from build123d import *

# Parameters (mm, degrees)
EXTRUDE_1_DEPTH     = 5
SKETCH_18_W         = 75
SKETCH_18_H         = 10
EXTRUDE_2_DEPTH     = 30
SKETCH_19_R         = 2.5
CUT_EXTRUDE_3_DEPTH = 85.889634232
EXTRUDE_3_DEPTH     = 10
SKETCH_21_R         = 2.5
CUT_EXTRUDE_4_DEPTH = 137.267200749


with BuildPart() as part:
    # ｽｹｯﾁ1 → ﾎﾞｽ - 押し出し1 (new body)
    with BuildSketch(Plane(origin=(0, 0, 0), x_dir=(1, 0, 0), z_dir=(0, 1, 0))):
        with BuildLine():
            Line((-37.5, 0), (-37.5, -70))
            Line((-37.5, -70), (37.5, -70))
            Line((37.5, -70), (37.5, 0))
            ThreePointArc((37.5, 0), (0, 37.5), (-37.5, 0))
        make_face()
    extrude(amount=EXTRUDE_1_DEPTH)

    # ｽｹｯﾁ18 → ﾎﾞｽ - 押し出し2 (add)
    with BuildSketch(Plane(origin=(0, 5, 0), x_dir=(1, 0, 0), z_dir=(0, 1, 0))):
        with Locations((0, -65)):
            Rectangle(SKETCH_18_W, SKETCH_18_H)
    extrude(amount=EXTRUDE_2_DEPTH)

    # ｽｹｯﾁ19 → ｶｯﾄ - 押し出し3 (cut, through all)
    with BuildSketch(Plane(origin=(0, 5, 0), x_dir=(1, 0, 0), z_dir=(0, 1, 0))):
        with Locations(Location((0, 31.5, 0), (0, 0, 270))):
            Circle(SKETCH_19_R)
        with Locations(Location((0, -31.5, 0), (0, 0, 90))):
            Circle(SKETCH_19_R)
    extrude(amount=-CUT_EXTRUDE_3_DEPTH, mode=Mode.SUBTRACT)

    # ｽｹｯﾁ20 → ﾎﾞｽ - 押し出し3 (add)
    with BuildSketch(Plane.XY.offset(70)):
        with BuildLine():
            Line((-37.5, 50), (-37.5, 35))
            Line((-37.5, 35), (37.5, 35))
            Line((37.5, 35), (37.5, 50))
            ThreePointArc((37.5, 50), (0, 87.5), (-37.5, 50))
        make_face()
    extrude(amount=-EXTRUDE_3_DEPTH)

    # ｽｹｯﾁ21 → ｶｯﾄ - 押し出し4 (cut, through all)
    with BuildSketch(Plane(origin=(0, 0, 60), x_dir=(-1, 0, 0), z_dir=(0, 0, -1))):
        with Locations((0, 81.5)):
            Circle(SKETCH_21_R)
        with Locations(Location((0, 18.5, 0), (0, 0, 180))):
            Circle(SKETCH_21_R)
    extrude(amount=-CUT_EXTRUDE_4_DEPTH, mode=Mode.SUBTRACT)


solid = part.part
Verification items for the finished model (mm, model axes). A direction names the side the tool comes from. Coordinates: 2 decimals unless noted, no trailing zeros. Write each loop counter-clockwise with the first axis right and the second up, starting at its lowest first coordinate (ties: lowest second). Pieces come first, ordered by that corner, then holes. Notation, with made-up numbers: (53, 66.25) -> (69, 66.25) arc R14 cw to (69, 89.25) -> close; hole circle Ø6 at (-37, 39.25). An arc over 180 degrees is marked (long way). One line per item, written item: value. Start each with the question number.
Q1. Mould release check, pull along Z, two halves, no side actions. Record for faces 1 (the cylindrical face through (0, 3, -34)), 2 (the flat face through (37.5, 4.5, 50.7)), 3 (the flat face through (-1, 44, 70)): pulls with the +Z half, pulls with the -Z half, needs draft (parallel to the pull), parting line crosses it, or undercut.
Q2. Cross-section at A-A on y = 18.5. Enter the section's corners in (x, z), and give its area (3 significant figures).
Q3. Thickness scan on L1, parallel to Y at x = 0, z = 65; L2, parallel to X at y = 18.5, z = 66.25; L3, parallel to Y at x = 25.5, z = 20. Record the ranges inside material, lowest first. Write a range as from..to.
Q4. Go/stop test with flat-tipped pins: P1, Ø5, axis at x = 21, z = 22.5, coming from the +Y side; P2, Ø2, axis at x = 10, y = 43, coming from the -Z side. Record where each tip stops, or that it passes through.
Q5. Access from +Z, -Z, +X, -X, +Y, -Y to the whole of each face (thin tool, end or side, straight path). Record for faces 4 (the flat face through (-1, 47, 60)), 5 (the flat face through (-37.5, 16, 64)).
Q6. Cross-section at B-B on x = 0. Enter the section's corners in (y, z).
Q7. Cross-section at C-C on z = 31.5. Enter the section's corners in (x, y), and give its area (3 significant figures).
Q8. Cross-section at D-D on y = 42. Enter the section's corners in (x, z).
Checked values:
1. face 1: undercut
1. face 2: needs draft
1. face 3: pulls with the +Z half
2. outline: (-37.5, 60) -> (-2.5, 60) -> (-2.5, 70) -> (-37.5, 70) -> close; (2.5, 60) -> (37.5, 60) -> (37.5, 70) -> (2.5, 70) -> close
2. area: 700 mm²
3. L1: y = 0..16, 21..79, 84..87.5
3. L2: x = -37.5..-2.5, 2.5..37.5
3. L3: y = 0..5
4. P1: stops at y = 5
4. P2: stops at z = 60
5. face 4: -Z, +X, -X, +Y
5. face 5: +Z, -Z, -X, +Y, -Y
6. outline: (0, -37.5) -> (5, -37.5) -> (5, -34) -> (0, -34) -> close; (0, -29) -> (5, -29) -> (5, 29) -> (0, 29) -> close; (0, 34) -> (5, 34) -> (5, 60) -> (16, 60) -> (16, 70) -> (0, 70) -> close; (21, 60) -> (79, 60) -> (79, 70) -> (21, 70) -> close; (84, 60) -> (87.5, 60) -> (87.5, 70) -> (84, 70) -> close
7. outline: (-37.5, 0) -> (-2.5, 0) -> (-2.5, 5) -> (-37.5, 5) -> close; (2.5, 0) -> (37.5, 0) -> (37.5, 5) -> (2.5, 5) -> close
7. area: 350 mm²
8. outline: (-37.5, 60) -> (37.5, 60) -> (37.5, 70) -> (-37.5, 70) -> close
